from build123d import *

# Parameters (mm, degrees)
SKETCH_1_W           = 210
SKETCH_1_H           = 230
EXTRUDE_1_DEPTH      = 6
SKETCH_2_W           = 9.85
SKETCH_2_H           = 209.85
SKETCH_2_W_2         = 10
EXTRUDE_3_DEPTH      = 15
SKETCH_3_R           = 2
CUT_EXTRUDE_1_DEPTH  = 10
SKETCH_17_W          = 6
SKETCH_17_H          = 230
EXTRUDE_9_DEPTH      = 66
EXTRUDE_10_DEPTH     = 6
CHAMFER_3_SIZE       = 8
SKETCH_19_W          = 5
SKETCH_19_H          = 230
EXTRUDE_11_DEPTH     = 66
FILLET_4_R           = 10
SKETCH_21_R          = 2.3
CUT_EXTRUDE_9_DEPTH  = 6
EXTRUDE_13_DEPTH     = 66
SKETCH_28_W          = 53
SKETCH_28_H          = 3
EXTRUDE_14_DEPTH     = 66
SKETCH_30_W          = 2
SKETCH_30_H          = 2
CUT_EXTRUDE_10_DEPTH = 30
SKETCH_31_R          = 1.25
SKETCH_31_W          = 13
SKETCH_31_H          = 13
CUT_EXTRUDE_11_DEPTH = 316.06185361
SKETCH_32_W          = 12
SKETCH_32_H          = 10
CUT_EXTRUDE_12_DEPTH = 320.662321834
CUT_EXTRUDE_13_REACH = 278.182
SKETCH_33_W          = 20
SKETCH_33_H          = 8.46
SKETCH_34_R          = 2.25
CUT_EXTRUDE_14_DEPTH = 30
SKETCH_36_R          = 2.25
CUT_EXTRUDE_15_DEPTH = 30


with BuildPart() as part:
    # 草图1 → 凸台-拉伸1 (new body)
    with BuildSketch(Plane.XY):
        with Locations((105, 115)):
            Rectangle(SKETCH_1_W, SKETCH_1_H)
    extrude(amount=EXTRUDE_1_DEPTH)

    # 草图2 → 凸台-拉伸3 (add)
    with BuildSketch(Plane(origin=(0, 0, 0), x_dir=(-1, 0, 0), z_dir=(0, 0, -1))):
        with Locations((-197, 115)):
            Rectangle(SKETCH_2_W, SKETCH_2_H)
        with Locations((-9.85, 115)):
            Rectangle(SKETCH_2_W_2, SKETCH_2_H)
    extrude(amount=EXTRUDE_3_DEPTH)

    # 草图3 → 切除-拉伸1 (cut)
    with BuildSketch(Plane(origin=(0, 0, 0), x_dir=(-1, 0, 0), z_dir=(0, 0, -1))):
        with Locations((-169.6425573, 192.25)):
            Circle(SKETCH_3_R)
        with Locations((-150.5, 205)):
            Circle(SKETCH_3_R)
        with Locations((-150.5, 179.5)):
            Circle(SKETCH_3_R)
        with Locations(Location((-150.5, 50.5, 0), (0, 0, 180))):
            Circle(SKETCH_3_R)
        with Locations(Location((-150.5, 25, 0), (0, 0, 180))):
            Circle(SKETCH_3_R)
        with Locations(Location((-169.6425573, 37.75, 0), (0, 0, 180))):
            Circle(SKETCH_3_R)
        with Locations((-34.3574427, 192.25)):
            Circle(SKETCH_3_R)
        with Locations((-53.5, 205)):
            Circle(SKETCH_3_R)
        with Locations((-53.5, 179.5)):
            Circle(SKETCH_3_R)
        with Locations(Location((-53.5, 50.5, 0), (0, 0, 180))):
            Circle(SKETCH_3_R)
        with Locations(Location((-53.5, 25, 0), (0, 0, 180))):
            Circle(SKETCH_3_R)
        with Locations(Location((-34.3574427, 37.75, 0), (0, 0, 180))):
            Circle(SKETCH_3_R)
    extrude(amount=-CUT_EXTRUDE_1_DEPTH, mode=Mode.SUBTRACT)

    # 草图17 → 凸台-拉伸9 (add)
    with BuildSketch(Plane.XY.offset(6)):
        with Locations((3, 115)):
            Rectangle(SKETCH_17_W, SKETCH_17_H)
        with Locations((207, 115)):
            Rectangle(SKETCH_17_W, SKETCH_17_H)
    extrude(amount=EXTRUDE_9_DEPTH)

    # 草图18 → 凸台-拉伸10 (add)
    with BuildSketch(Plane.XY.offset(72)):
        Polygon((210, 230), (204, 230), (6, 230), (0, 230), (0, 0), (6, 0), (204, 0), (210, 0), align=None)
    extrude(amount=EXTRUDE_10_DEPTH)

    # 倒角3
    chamfer_3_edges = [part.edges().sort_by_distance(p)[0] for p in [
        (210, 115, 78),
        (0, 115, 78),
    ]]
    chamfer(chamfer_3_edges, length=CHAMFER_3_SIZE)

    # 草图19 → 凸台-拉伸11 (add)
    with BuildSketch(Plane(origin=(0, 0, 72), x_dir=(-1, 0, 0), z_dir=(0, 0, -1))):
        with Locations((-134, 115)):
            Rectangle(SKETCH_19_W, SKETCH_19_H)
        with Locations((-76, 115)):
            Rectangle(SKETCH_19_W, SKETCH_19_H)
    extrude(amount=EXTRUDE_11_DEPTH)

    # 圆角4
    fillet_4_edges = [part.edges().sort_by_distance(p)[0] for p in [
        (6, 115, 6),
        (6, 115, 72),
        (204, 115, 6),
        (204, 115, 72),
        (73.5, 115, 6),
        (73.5, 115, 72),
        (136.5, 115, 72),
        (136.5, 115, 6),
    ]]
    fillet(fillet_4_edges, radius=FILLET_4_R)

    # 草图21 → 切除-拉伸9 (cut)
    with BuildSketch(Plane.XY.offset(72)):
        with Locations((105, 130)):
            Circle(SKETCH_21_R)
        with Locations((105, 100)):
            Circle(SKETCH_21_R)
    extrude(amount=CUT_EXTRUDE_9_DEPTH, mode=Mode.SUBTRACT)

    # 草图26 → 凸台-拉伸13 (add)
    with BuildSketch(Plane(origin=(0, 0, 72), x_dir=(-1, 0, 0), z_dir=(0, 0, -1))):
        with BuildLine():
            Line((-131.26, 181), (-131.26, 179))
            ThreePointArc((-131.26, 179), (-131.5, 178.76), (-131.74, 179))
            Line((-131.74, 179), (-131.74, 181))
            ThreePointArc((-131.74, 181), (-131.5, 181.24), (-131.26, 181))
        make_face()
        with BuildLine():
            Line((-131.26, 22.5), (-131.26, 20.5))
            ThreePointArc((-131.26, 20.5), (-131.5, 20.26), (-131.74, 20.5))
            Line((-131.74, 20.5), (-131.74, 22.5))
            ThreePointArc((-131.74, 22.5), (-131.5, 22.74), (-131.26, 22.5))
        make_face()
    extrude_13 = extrude(amount=EXTRUDE_13_DEPTH)

    # 镜向2: 凸台-拉伸13 across plane
    add(extrude_13.mirror(Plane.ZY.offset(-105)))

    # 草图28 → 凸台-拉伸14 (add)
    with BuildSketch(Plane(origin=(0, 0, 72), x_dir=(-1, 0, 0), z_dir=(0, 0, -1))):
        with Locations((-105, 9.96)):
            Rectangle(SKETCH_28_W, SKETCH_28_H)
    extrude(amount=EXTRUDE_14_DEPTH)

    # 草图30 → 切除-拉伸10 (cut)
    with BuildSketch(Plane(origin=(0, 230, 0), x_dir=(1, 0, 0), z_dir=(0, 1, 0))):
        with Locations((77.5, -37)):
            Rectangle(SKETCH_30_W, SKETCH_30_H)
    extrude(amount=-CUT_EXTRUDE_10_DEPTH, mode=Mode.SUBTRACT)

    # 草图31 → 切除-拉伸11 (cut, through all)
    with BuildSketch(Plane.XZ.offset(-8.46)):
        with Locations((92.7, 15.7)):
            Circle(SKETCH_31_R)
        with Locations((117.3, 15.7)):
            Circle(SKETCH_31_R)
        with Locations((105, 15.7)):
            Rectangle(SKETCH_31_W, SKETCH_31_H)
    extrude(amount=-CUT_EXTRUDE_11_DEPTH, mode=Mode.SUBTRACT)

    # 草图32 → 切除-拉伸12 (cut, through all)
    with BuildSketch(Plane.XY.offset(6)):
        with Locations((125.5, 3.46)):
            Rectangle(SKETCH_32_W, SKETCH_32_H)
    extrude(amount=-CUT_EXTRUDE_12_DEPTH, mode=Mode.SUBTRACT)

    # 草图33 → 切除-拉伸13 (cut, up to next)
    with BuildSketch(Plane.ZY.offset(-131.5), mode=Mode.PRIVATE) as cut_extrude_13_sk1:
        with Locations((40, 4.23)):
            Rectangle(SKETCH_33_W, SKETCH_33_H)
    cut_extrude_13_tool1 = extrude(cut_extrude_13_sk1.sketch, amount=-CUT_EXTRUDE_13_REACH, mode=Mode.PRIVATE) & part.part
    add(cut_extrude_13_tool1.solids().sort_by_distance((131.5, 4.23, 40))[0], mode=Mode.SUBTRACT)

    # 草图34 → 切除-拉伸14 (cut)
    with BuildSketch(Plane(origin=(0, 0, 72), x_dir=(-1, 0, 0), z_dir=(0, 0, -1))):
        with Locations((-185.25, 115)):
            Circle(SKETCH_34_R)
        with Locations((-155.25, 115)):
            Circle(SKETCH_34_R)
    extrude(amount=-CUT_EXTRUDE_14_DEPTH, mode=Mode.SUBTRACT)

    # 草图36 → 切除-拉伸15 (cut)
    with BuildSketch(Plane(origin=(0, 0, 72), x_dir=(-1, 0, 0), z_dir=(0, 0, -1))):
        with Locations((-54.75, 115)):
            Circle(SKETCH_36_R)
        with Locations((-24.75, 115)):
            Circle(SKETCH_36_R)
    extrude(amount=-CUT_EXTRUDE_15_DEPTH, mode=Mode.SUBTRACT)


solid = part.part
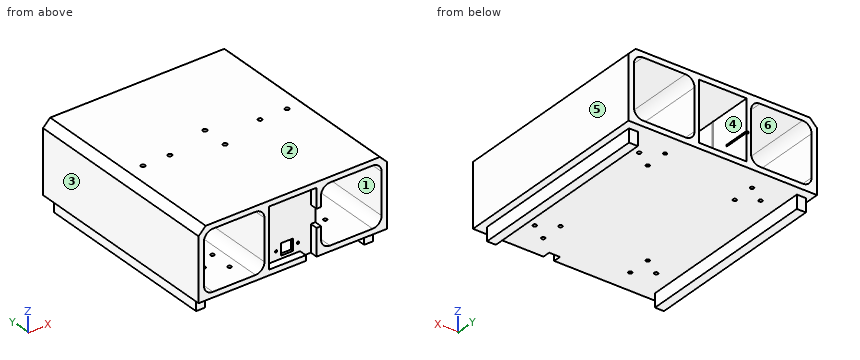
Geometry: final body of the model. Coordinates: model frame, mm. Face numbers are marked on the shaded views. A direction names the side the tool comes from. Coordinates: 2 decimals unless noted, no trailing zeros.
1) Draft query along Z for the marked faces 1, 2 and 3. Return one class per face: released by +Z, released by -Z, zero draft, split by the parting line, or undercut.
Result sheet:
face 1: undercut
face 2: released by +Z
face 3: zero draft
2) Ray query, probe 1 along Y at (x, z) = (150, 2); probe 2 along X at (y, z) = (133, 59.5); probe 3 along X at (y, z) = (179.5, 4.1). Return the intervals inside material, ascending.
Result sheet:
probe 1: y = 0 to 23.06, 26.94 to 48.56, 52.44 to 177.56, 181.44 to 203.06, 206.94 to 230
probe 2: x = 0 to 6, 73.5 to 78.5, 131.5 to 136.5, 204 to 210
probe 3: x = 0 to 51.5, 55.5 to 148.5, 152.5 to 210
3) Set-up query: the marked faces 4, 5 and 6. Return all of +Z, -Z, +X, -X, +Y, -Y with unobstructed straight access to the full face (end or side cutting, diameter ignored); none if empty.
Result sheet:
face 4: +Y
face 5: +Z, -Z, +X, +Y, -Y
face 6: +Y, -Y
4) First-contact query: P1, Ø16, axis at x = 115.5, y = 149, coming from the -Z side; P2, Ø3.5, axis at x = 150.5, y = 25, coming from the -Z side; P3, Ø4.5, axis at y = 80.5, z = -5.5, coming from the -X side. Flat tips, straight axial feed; report the tip coordinate or a pass-through.
Result sheet:
P1: stops at z = 0
P2: stops at z = 72
P3: stops at x = 4.85
5) Section A-A (y = 92). Give the number of separate pieces and of enclosed holes in the cut face, then the cut area to 3 significant figures.
Result sheet:
separate pieces: 1
enclosed holes: 3
area: 4,380 mm2
